Here's how the part is built. I have some questions about the finished solid (model axes, mm). A direction names the side the tool comes from. Give positions to 0.01 mm unless a question says otherwise; leave off trailing zeros. Order: outer loops, then holes, each group sorted by start corner. A loop starts at its lowest first (then second) coordinate and runs counter-clockwise, first axis right, second up.
Autodesk Inventor part; units mm, degrees
ref_plane "YZ Plane" through (0, 0, 0) normal (1, 0, 0) x (0, 1, 0)
ref_plane "XZ Plane" through (0, 0, 0) normal (0, 1, 0) x (-1, 0, 0)
ref_plane "XY Plane" through (0, 0, 0) normal (0, 0, 1) x (1, 0, 0)
sketch "スケッチ1" plane through (0, 0, 0) normal (0, 1, 0) x (-1, 0, 0)
  line L0 (0, 0) -> (120, 0)
  line L1 (120, 0) -> (120, -140)
  line L2 (120, -140) -> (0, -140)
  line L3 (0, -140) -> (0, 0)
  dimension "d0" = 120
  dimension "d1" = 140
extrude "押し出し1" add sketch "スケッチ1" along normal blind 3
sketch "スケッチ2" plane through (0, 3, 0) normal (0, 1, 0) x (1, 0, 0)
  line L0 (-120, 140) -> (-120, 0)
  line L1 (0, 140) -> (-120, 140)
  line L2 (-120, 0) -> (0, 140)
  circle A0 centre (-60, 70) radius 49
  line L3 (-120, 70) -> (0, 70)
  line L4 (0, 0) -> (0, 140)
  line L5 (-60, 70) -> (-14.7299, 88.7515)
  point P0 (-41.2485, 115.2701)
  point P1 (-78.7515, 115.2701)
  point P2 (-105.2701, 88.7515)
  point P3 (-105.2701, 51.2485)
  point P4 (-78.7515, 24.7299)
  point P5 (-41.2485, 24.7299)
  point P6 (-14.7299, 51.2485)
  dimension "d4" = 98
  dimension "d5" = 22.5
  dimension "d8" = 360
hole "穴1" at (-14.7299, 3, -88.7515) at (-41.2485, 3, -115.2701) at (-78.7515, 3, -115.2701) at (-105.2701, 3, -88.7515) at (-105.2701, 3, -51.2485) at (-78.7515, 3, -24.7299) at (-41.2485, 3, -24.7299) at (-14.7299, 3, -51.2485) direction (0, -1, 0) diameter 4.2 end through all
sketch "スケッチ3" plane through (0, 3, 0) normal (0, 1, 0) x (1, 0, 0)
  line L0 (-120, 140) -> (-120, 0)
  line L1 (0, 140) -> (-120, 140)
  line L2 (-120, 0) -> (0, 140)
  circle A0 centre (-60, 70) radius 40.5
  line L3 (-120, 0) -> (0, 0)
  line L4 (-99, 0) -> (-99, 140)
  line L5 (-21, 0) -> (-21, 140)
  point P0 (-21, 70)
  point P1 (-99, 80.9202)
  point P2 (-99, 59.0798)
  point P3 (-21, 59.0798)
  point P4 (-21, 80.9202)
  dimension "d17" = 81
  dimension "d20" = 39
  dimension "d21" = 39
extrude "押し出し2" cut sketch "スケッチ3" against normal blind 3 contours A0 L2 L4 | L2 A0 L5 picked at (-76.2281, 82.7678) picked at (-47.1316, 53.0288)
sketch "スケッチ4" plane through (0, 3, 0) normal (0, 1, 0) x (1, 0, 0)
  line L0 (-120, 140) -> (-120, 0)
  line L1 (-120, 5) -> (0, 5)
  line L2 (0, 0) -> (0, 140)
  line L3 (-120, 135) -> (0, 135)
  line L4 (-120, 0) -> (0, 0)
  line L5 (0, 140) -> (-120, 140)
  line L6 (-120, 0) -> (0, 0)
  line L7 (-115, 0) -> (-115, 140)
  line L8 (-5, 140) -> (-5, 0)
  point P0 (-115, 5)
  point P1 (-5, 5)
  point P2 (-5, 135)
  point P3 (-115, 135)
  dimension "d22" = 5
  dimension "d23" = 5
  dimension "d24" = 5
  dimension "d25" = 5
hole "穴2" at (-115, 3, -5) at (-5, 3, -5) at (-5, 3, -135) at (-115, 3, -135) direction (0, -1, 0) diameter 3.2 end through all
equation "\"d15\" = Thickness"
equation "\"BendRadius\" = Thickness"
equation "\"BendReliefWidth\" = Thickness"
equation "\"BendReliefDepth\" = 0.5 * Thickness"
equation "\"CornerReliefSize\" = 4 * Thickness"
equation "\"MinimumRemnant\" = 2 * Thickness"
equation "\"TransitionRadius\" = BendRadius"
equation "\"JacobiRadiusSize\" = BendRadius"
equation "\"GapSize\" = Thickness"
properties part number "base_plate2" material "アルミニウム 6061"
Q1. If we section it at D-D on x = -53: List the corners of the cut face in (y, z) for me.
Filled sheet:
outline: (0, -140) - (3, -140) - (3, -109.89) - (0, -109.89) - close; (0, -30.11) - (3, -30.11) - (3, 0) - (0, 0) - close
Q2. I need wall thicknesses on L1, parallel to Z at x = -115, y = 2.1; L2, parallel to Z at x = -105, y = 1; L3, parallel to X at y = 2.3, z = -65. Which ranges of each line are inside material? Lowest first, please.
Filled sheet:
L1: z = -140 to -136.6, -133.4 to -6.6, -3.4 to 0
L2: z = -140 to -90.83, -86.67 to -53.33, -49.17 to 0
L3: x = -120 to -99, -21 to 0
Q3. For faces 1 (the face through (-120, 1, -69)), 2 (the face through (-59.264, 1.521, -110.493)), which set-ups out of +Z, -Z, +X, -X, +Y, -Y let a thin tool reach every point of the face, with its end or its side?
Filled sheet:
face 1: +Z, -Z, -X, +Y, -Y
face 2: +Y, -Y
Q4. If we section it at A-A on z = -62: List the corners of the cut face in (x, y) for me.
Filled sheet:
outline: (-120, 0) - (-99, 0) - (-99, 3) - (-120, 3) - close; (-21, 0) - (0, 0) - (0, 3) - (-21, 3) - close
Q5. I'm going to push a flat-ended pin straight in: P1, Ø2.5, axis at x = -115, z = -135, coming from the -Y side. Where does the tip first touch, or does it pass through?
Filled sheet:
P1: passes through
Q6. Thinking about a two-plate mould opening in X: for faces 3 (the face through (0, 1, -71)), 4 (the face through (-42.668, 1.479, -116.818)), 5 (the face through (-19, 0, -69)), which applies, released by +X, released by -X, zero draft, split by the parting line, or undercut?
Filled sheet:
face 3: released by +X
face 4: undercut
face 5: zero draft
Q7. If we section it at C-C on z = -135: List the corners of the cut face in (x, y) for me.
Filled sheet:
outline: (-120, 0) - (-116.6, 0) - (-116.6, 3) - (-120, 3) - close; (-113.4, 0) - (-6.6, 0) - (-6.6, 3) - (-113.4, 3) - close; (-3.4, 0) - (0, 0) - (0, 3) - (-3.4, 3) - close
Q8. If we section it at B-B on x = -5: List the corners of the cut face in (y, z) for me.
Filled sheet:
outline: (0, -140) - (3, -140) - (3, -136.6) - (0, -136.6) - close; (0, -133.4) - (3, -133.4) - (3, -6.6) - (0, -6.6) - close; (0, -3.4) - (3, -3.4) - (3, 0) - (0, 0) - close
